```python
from build123d import *

# Parameters (mm, degrees)
SKETCH1_W           = 16
SKETCH1_H           = 13
BOSS_EXTRUDE1_DEPTH = 1
SKETCH2_R           = 1.5
BOSS_EXTRUDE2_DEPTH = 1


with BuildPart() as part:
    # Sketch1 → Boss-Extrude1 (new body, symmetric)
    with BuildSketch(Plane.XY):
        Rectangle(SKETCH1_W, SKETCH1_H)
    extrude(amount=BOSS_EXTRUDE1_DEPTH, both=True)

    # Sketch2 → Boss-Extrude2 (add, symmetric)
    with BuildSketch(Plane.XY):
        with BuildLine():
            Line((-9.75, 2.75), (-8, 2.75))
            Line((-8, 2.75), (-8, -2.75))
            Line((-8, -2.75), (-9.75, -2.75))
            ThreePointArc((-9.75, -2.75), (-12.5, 0), (-9.75, 2.75))
        make_face()
        with Locations((-9.75, 0)):
            Circle(SKETCH2_R, mode=Mode.SUBTRACT)
        with BuildLine():
            Line((9.75, -2.75), (8, -2.75))
            Line((8, -2.75), (8, 2.75))
            Line((8, 2.75), (9.75, 2.75))
            ThreePointArc((9.75, 2.75), (12.5, 0), (9.75, -2.75))
        make_face()
        with Locations((9.75, 0)):
            Circle(SKETCH2_R, mode=Mode.SUBTRACT)
    extrude(amount=BOSS_EXTRUDE2_DEPTH, both=True)


solid = part.part
```
Here's how the part is built. I have some questions about the finished solid (model axes, mm). A direction names the side the tool comes from. Give positions to 0.01 mm unless a question says otherwise; leave off trailing zeros. Write each loop counter-clockwise with the first axis right and the second up, starting at its lowest first coordinate (ties: lowest second). Pieces come first, ordered by that corner, then holes. Notation, with made-up numbers: M 80.5,13.5 L 110.5,13.5 A10 ccw 110.5,29.5 Z; hole C 2,64.25 d1. An arc over 180 degrees is marked long. Put each result on its own line as item: value. Start each with the question number.
Item 1: If we section it at C-C, the plane z = 0.65: Write out the boundary of the cut face in (x, y), then the cut area to 3 significant figures.
Item 2: Thinking about a two-plate mould opening in X: for faces 1 (the cylindrical face through (8.25, 0.07, -0.01)), 2 (the cylindrical face through (-11.25, 0.07, -0.01)), 3 (the flat face through (8, -5, 0)), 4 (the flat face through (0, 6.5, 0)), which applies, +X half, -X half, draft (parallel to the pull), parting line (faces both ways), or undercut?
Item 3: Will these pins go through, and if not, where does the flat tip stop? pin 1 (0.5 mm diameter, centred on x = -8.5, z = 0.5, fed in from -Y); pin 2 (0.5 mm diameter, centred on x = -9, z = -0.5, fed in from +Y); pin 3 (0.6 mm diameter, centred on y = -4, z = -0.5, fed in from -X).
Item 4: If we section it at B-B, the plane x = 9: Write out the boundary of the cut face in (y, z).
Item 5: On a 3-axis mill with a long thin cutter (end or side, diameter ignored), from which of +Z, -Z, +X, -X, +Y, -Y can I reach the whole of each face in a straight line? I mean faces 5 (the flat face through (0, 0, -1)), 6 (the flat face through (-9, 2.75, 0)), 7 (the flat face through (8, 5, 0)), 8 (the flat face through (-9, -2.75, 0)), 9 (the flat face through (9, -2.75, 0)). Say none if no direction works.
Item 6: I need wall thicknesses on L1, parallel to Y at x = -9.75, z = 0; L2, parallel to X at y = 3.25, z = 0.55; L3, parallel to X at y = -0.5, z = -0.25. Which ranges of each line are inside material? Lowest first, please. Write a range as from..to.
Item 7: If we section it at D-D, the plane y = 5.5: Write out the boundary of the cut face in (x, z), then the cut area to 3 significant figures.
Item 8: If we section it at A-A, the plane y = 0: Write out the boundary of the cut face in (x, z).
Values:
1. outline: M -9.75,-2.75 L -8,-2.75 L -8,-6.5 L 8,-6.5 L 8,-2.75 L 9.75,-2.75 A2.75 ccw 9.75,2.75 L 8,2.75 L 8,6.5 L -8,6.5 L -8,2.75 L -9.75,2.75 A2.75 ccw Z; hole C -9.75,0 d3; hole C 9.75,0 d3
1. area: 237 mm²
2. face 1: undercut
2. face 2: undercut
2. face 3: +X half
2. face 4: draft
3. pin 1: y = -2.75
3. pin 2: y = 2.75
3. pin 3: x = -8
4. outline: M -2.75,-1 L -1.3,-1 L -1.3,1 L -2.75,1 Z; M 1.3,-1 L 2.75,-1 L 2.75,1 L 1.3,1 Z
5. face 5: -Z, +X, -X, +Y, -Y
5. face 6: +Z, -Z, -X, +Y
5. face 7: +Z, -Z, +X, +Y
5. face 8: +Z, -Z, -X, -Y
5. face 9: +Z, -Z, +X, -Y
6. L1: -2.75..-1.5, 1.5..2.75
6. L2: -8..8
6. L3: -12.45..-11.16, -8.34..8.34, 11.16..12.45
7. outline: M -8,-1 L 8,-1 L 8,1 L -8,1 Z
7. area: 32.0 mm²
8. outline: M -12.5,-1 L -11.25,-1 L -11.25,1 L -12.5,1 Z; M -8.25,-1 L 8.25,-1 L 8.25,1 L -8.25,1 Z; M 11.25,-1 L 12.5,-1 L 12.5,1 L 11.25,1 Z
